from build123d import *

# Parameters (mm, degrees)
SKETCH1_R               = 10
BOSS_EXTRUDE1_DEPTH     = 3
SKETCH2_R               = 5
BOSS_EXTRUDE2_DEPTH     = 10.5
CUT_EXTRUDE1_DEPTH      = 20.551214796
CUT_EXTRUDE1_DEPTH_BACK = 20.551214796
SKETCH3_R               = 2.5
CHAMFER1_SIZE           = 0.25
CUT_EXTRUDE2_DEPTH      = 20.551214796
CUT_EXTRUDE2_DEPTH_BACK = 20.551214796
SKETCH4_R               = 1.5


with BuildPart() as part:
    # Sketch1 → Boss-Extrude1 (new body)
    with BuildSketch(Plane.XY):
        Circle(SKETCH1_R)
    extrude(amount=BOSS_EXTRUDE1_DEPTH)

    # Sketch2 → Boss-Extrude2 (add)
    with BuildSketch(Plane.XY.offset(3)):
        with Locations(Location((0, 0, 0), (0, 0, 180))):
            Circle(SKETCH2_R)
    extrude(amount=BOSS_EXTRUDE2_DEPTH)

    # Sketch3 → Cut-Extrude1 (cut, two sides: drawn at the far end of the back side and taken through both)
    with BuildSketch(Plane.XY.offset(13.5).offset(-CUT_EXTRUDE1_DEPTH_BACK)):
        Circle(SKETCH3_R)
    extrude(amount=CUT_EXTRUDE1_DEPTH + CUT_EXTRUDE1_DEPTH_BACK, mode=Mode.SUBTRACT)

    # Chamfer1
    chamfer1_edges = [part.edges().sort_by_distance(p)[0] for p in [
        (-10, 0, 0),
        (-10, 0, 3),
        (5, 0, 3),
        (5, 0, 13.5),
    ]]
    chamfer(chamfer1_edges, length=CHAMFER1_SIZE)

    # Sketch4 → Cut-Extrude2 (cut, two sides: drawn at the far end of the back side and taken through both)
    with BuildSketch(Plane(origin=(0, 0, 0), x_dir=(-1, 0, 0), z_dir=(0, 0, -1)).offset(-CUT_EXTRUDE2_DEPTH_BACK)):
        with Locations((-5.303300859, 5.303300859)):
            Circle(SKETCH4_R)
        with Locations((5.303300859, 5.303300859)):
            Circle(SKETCH4_R)
        with Locations((5.303300859, -5.303300859)):
            Circle(SKETCH4_R)
        with Locations((-5.303300859, -5.303300859)):
            Circle(SKETCH4_R)
    extrude(amount=CUT_EXTRUDE2_DEPTH + CUT_EXTRUDE2_DEPTH_BACK, mode=Mode.SUBTRACT)


solid = part.part
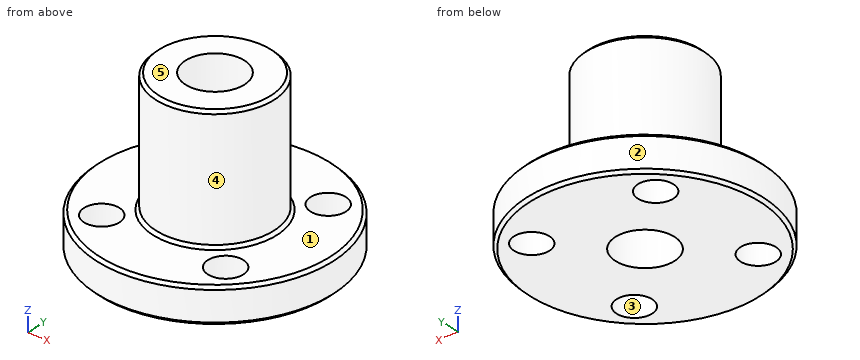
Part model, mm, in its own coordinate system. Face numbers are marked on the shaded views. A direction names the side the tool comes from. Round coordinates to 2 decimals unless told otherwise and drop trailing zeros. Write each loop counter-clockwise with the first axis right and the second up, starting at its lowest first coordinate (ties: lowest second). Pieces come first, ordered by that corner, then holes. Notation, with made-up numbers: M 49,47.25 L 58,47.25 A19 ccw 58,53.25 Z; hole C 36,-8.5 d9. An arc over 180 degrees is marked long. Return JSON: item names as keys, results as strings. Group by question number.
(1) Which spindle directions (+Z, -Z, +X, -X, +Y, -Y) get a long thin tool onto all of the face, cutting with end or side? Do the marked faces 4 and 5. Say none if no direction does.
(2) Two-plate mould, pull along X, no slides. Class the marked faces 1, 2 and 3: +X half, -X half, draft (parallel to the pull), parting line (faces both ways), or undercut.
(3) Saw through at A-A on x = 0. Write the cut outline in (y, z), then the cut area to 3 significant figures.
(4) Drill centre lines: probe 1 along Y at (x, z) = (0, 7.25); probe 2 along Z at (x, y) = (-4, 4.25); probe 3 along Y at (x, z) = (-1, 1.5). Where is each one in solid material? Low to high.
(5) Pin check, flat tips, straight feed: pin 1 Ø1 at (x, z) = (-2, 4) entering from +Y; pin 2 Ø2 at (x, z) = (-5.5, 10.5) entering from +Y; pin 3 Ø4 at (x, y) = (4, 7.5) entering from +Z. Stop position of each tip, or through.
(6) Saw through at C-C on z = 5. Write the cut outline in (x, y), then the cut area to 3 significant figures.
(7) Saw through at D-D on x = -6.25. Count the separate pieces of the cut face and the enclosed holes in it, then the cut area to 3 significant figures.
Returned:
{
 "1": {"face 4": "+Z", "face 5": "+Z, +X, -X, +Y, -Y"},
 "2": {"face 1": "draft", "face 2": "parting line", "face 3": "undercut"},
 "3": {"outline": "M -10,0.25 L -9.75,0 L -2.5,0 L -2.5,13.5 L -4.75,13.5 L -5,13.25 L -5,3.25 L -5.25,3 L -9.75,3 L -10,2.75 Z; M 2.5,0 L 9.75,0 L 10,0.25 L 10,2.75 L 9.75,3 L 5.25,3 L 5,3.25 L 5,13.25 L 4.75,13.5 L 2.5,13.5 Z", "area": "97.4 mm²"},
 "4": {"probe 1": "-5 to -2.5, 2.5 to 5", "probe 2": "0 to 3", "probe 3": "-9.95 to -2.29, 2.29 to 9.95"},
 "5": {"pin 1": "y = 4.77", "pin 2": "y = 2.18", "pin 3": "z = 3"},
 "6": {"outline": "C 0,0 d10; hole C 0,0 d5", "area": "58.9 mm²"},
 "7": {"separate pieces": "3", "enclosed holes": "0", "area": "32.7 mm²"}
}
